```python
from build123d import *

# Parameters (mm, degrees)
PAD021_DEPTH         = 50
SKETCH042_R          = 45.5
PAD022_DEPTH         = 200
SKETCH043_R          = 41
SKETCH043_R_2        = 15
POCKET025_DEPTH      = 138
POCKET026_START      = -141
SKETCH044_R          = 47.5
SKETCH044_R_2        = 43
POCKET026_DEPTH      = 2
POCKET027_START      = -136
POCKET027_DEPTH      = 2
POCKET028_START      = -55
POCKET028_DEPTH      = 3
SKETCH049_R          = 30
POCKET030_DEPTH      = 110
POCKET031_START      = -61
POCKET031_DEPTH      = 2
SKETCH052_R          = 11
POCKET032_DEPTH      = 130
POCKET032_DEPTH_BACK = 5


with BuildPart() as body070:
    # Sketch041 → Pad021 (new body, symmetric)
    with BuildSketch(Plane.XY):
        Polygon((-45.5, 147), (45.5, 147), (45.5, 51), (0, 51), (-45.5, 51), align=None)
    extrude(amount=PAD021_DEPTH, both=True)


with BuildPart() as body071:
    # Sketch042 → Pad022 (new body)
    with BuildSketch(Plane.XZ):
        Circle(SKETCH042_R)
    extrude(amount=-PAD022_DEPTH)

    # Boolean004: intersect Body070
    add(body070.part, mode=Mode.INTERSECT)

    # Sketch043 → Pocket025 (cut)
    with BuildSketch(Plane.XZ):
        Circle(SKETCH043_R)
        Circle(SKETCH043_R_2, mode=Mode.SUBTRACT)
    extrude(amount=-POCKET025_DEPTH, mode=Mode.SUBTRACT)

    # Sketch044 → Pocket026 (cut)
    with BuildSketch(Plane.XZ.offset(POCKET026_START)):
        Circle(SKETCH044_R)
        Circle(SKETCH044_R_2, mode=Mode.SUBTRACT)
    extrude(amount=-POCKET026_DEPTH, mode=Mode.SUBTRACT)

    # Sketch044 → Pocket027 (cut)
    with BuildSketch(Plane.XZ.offset(POCKET027_START)):
        Circle(SKETCH044_R)
        Circle(SKETCH044_R_2, mode=Mode.SUBTRACT)
    extrude(amount=-POCKET027_DEPTH, mode=Mode.SUBTRACT)

    # Sketch044 → Pocket028 (cut)
    with BuildSketch(Plane.XZ.offset(POCKET028_START)):
        Circle(SKETCH044_R)
        Circle(SKETCH044_R_2, mode=Mode.SUBTRACT)
    extrude(amount=-POCKET028_DEPTH, mode=Mode.SUBTRACT)

    # Sketch049 → Pocket030 (cut)
    with BuildSketch(Plane.XZ):
        Circle(SKETCH049_R)
    extrude(amount=-POCKET030_DEPTH, mode=Mode.SUBTRACT)

    # Sketch044 → Pocket031 (cut)
    with BuildSketch(Plane.XZ.offset(POCKET031_START)):
        Circle(SKETCH044_R)
        Circle(SKETCH044_R_2, mode=Mode.SUBTRACT)
    extrude(amount=-POCKET031_DEPTH, mode=Mode.SUBTRACT)

    # Sketch052 → Pocket032 (cut, two sides)
    with BuildSketch(Plane.XZ) as pocket032_sk:
        Circle(SKETCH052_R)
    extrude(amount=-POCKET032_DEPTH, mode=Mode.SUBTRACT)
    extrude(pocket032_sk.sketch, amount=POCKET032_DEPTH_BACK, mode=Mode.SUBTRACT)


solid = body071.part
```
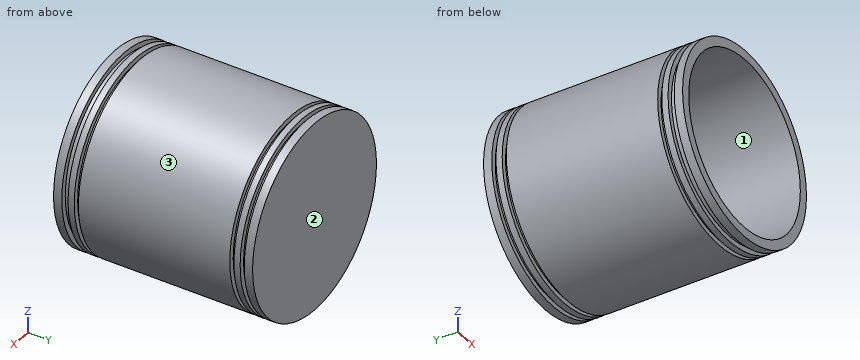
Here's how the part is built. I have some questions about the finished solid (model axes, mm). Face numbers are marked on the shaded views. Give positions to 0.01 mm unless a question says otherwise; leave off trailing zeros. Order: outer loops, then holes, each group sorted by start corner. A loop starts at its lowest first (then second) coordinate and runs counter-clockwise, first axis right, second up. Notation, with made-up numbers: M 58.5,-9 L 112.5,-9 A21 cw 112.5,21 Z; hole C 34,21 d1. An arc over 180 degrees is marked long. Use a Markdown table: item, result. Add a question column.
1. If we mould it in two halves opening along X, with no side actions, what happens to the marked faces 1, 2 and 3? For each: +X half, -X half, draft (parallel to the pull), parting line (faces both ways), or undercut.
2. I need wall thicknesses on probe 1 along Z at (x, y) = (0, 118); probe 2 along Z at (x, y) = (0, 71); probe 3 along Y at (x, z) = (36.5, 23). Which ranges of each line are inside material? Lowest first, please. Write a range as from..to.
3. Suppose I cut it at A-A (y = 121). List the corners of the cut face in (x, z) for me.
4. Suppose I cut it at B-B (y = 86). List the corners of the cut face in (x, z) for me.
5. For pin 1 Ø6.5 at (x, z) = (2, -1) entering from -Y; pin 2 Ø4 at (y, z) = (109.5, -15.5) entering from -X; pin 3 Ø12 at (y, z) = (74, 29.5) entering from -X, each with a flat end and sliding along its axis, tell me the tip position at first contact or that it passes through.
Results list:
| question | item | result |
|---|---|---|
| 1 | face 1 | undercut |
| 1 | face 2 | draft |
| 1 | face 3 | parting line |
| 2 | probe 1 | z = -45.5..-41, -15..-11, 11..15, 41..45.5 |
| 2 | probe 2 | z = -45.5..-41, 41..45.5 |
| 2 | probe 3 | y = 51..55, 58..61, 63..136, 138..141, 143..147 |
| 3 | outline | C 0,0 d91; C 0,0 d30; hole C 0,0 d82; hole C 0,0 d22 |
| 4 | outline | C 0,0 d91; hole C 0,0 d82 |
| 5 | pin 1 | stops at y = 130 |
| 5 | pin 2 | stops at x = -43.45 |
| 5 | pin 3 | stops at x = -38.96 |
